Geometry check sheet. Reference: the model listing, model coordinates, mm. A direction names the side the tool comes from. Coordinates: 2 decimals unless noted, no trailing zeros.
Autodesk Inventor part; units mm, degrees
ref_plane "YZ Plane" through (0, 0, 0) normal (1, 0, 0) x (0, 1, 0)
ref_plane "XZ Plane" through (0, 0, 0) normal (0, 1, 0) x (-1, 0, 0)
ref_plane "XY Plane" through (0, 0, 0) normal (0, 0, 1) x (1, 0, 0)
sketch "Эскиз1" plane through (0, 0, 0) normal (0, 0, 1) x (1, 0, 0)
  line L0 (0, 20) -> (0, 30)
  line L1 (1, 30.1228) -> (1, 72.3772)
  line L2 (0, 72.5) -> (0, 84.4165)
  line L3 (0, 84.4165) -> (15, 84.4165)
  line L4 (6, 71.3949) -> (6, 31.1051)
  line L5 (15, 20) -> (0, 20)
  line L6 (15, 30) -> (15, 20)
  line L7 (-3, 0) -> (18, 0) construction
  line L8 (0, -16.8833) -> (0, 101.2998) construction
  line L9 (15, 84.4165) -> (15, 72.5)
  line L10 (15, 72.5) -> (6, 71.3949)
  line L11 (15, 30) -> (6, 31.1051)
  line L12 (0, 30) -> (1, 30.1228)
  line L13 (0, 72.5) -> (1, 72.3772)
  point P0 (0, 0)
  point P1 (1, 77.4165)
  point P2 (7, 77.4165)
  point P3 (7, 28)
  dimension "d0" = 15
  dimension "d2" = 5
  dimension "d5" = 40
  dimension "d7" = 168.833
  dimension "d9" = 0
  dimension "d17" = 83
  dimension "d18" = 83
  dimension "d19" = 60
  dimension "d20" = 83
  dimension "d21" = 83
  dimension "d22" = 2
  dimension "d43" = 145
revolve "Вращение1" add sketch "Эскиз1" angle 360 about axis through (-10, 0, 0) along (1, 0, 0)
chamfer "Фаска1" distance 1 angle 45 2 edges at (15, -20, 0) (0, -20, 0)
fillet "Сопряжение3" radius 6 2 edges at (6, -71.3949, 0) (6, -31.1051, 0)
chamfer "Фаска2" distance 1 angle 45 1 edges at (15, -72.5, 0)
fillet "Сопряжение4" radius 6 2 edges at (1, -30.1228, 0) (1, -72.3772, 0)
chamfer "Фаска4" distance 0.5 angle 45 2 edges at (0, -84.4165, 0) (15, -84.4165, 0)
sketch "Эскиз2" plane through (15, 0, 0) normal (1, 0, 0) x (0, 0, -1)
  circle A0 centre (0, 0) radius 84.4165
  circle A1 centre (0, 0) radius 73.5
  circle A2 centre (0, 0) radius 84.4165
  line L0 (-84.4161, 0.25) -> (-78.79, 0.25)
  line L1 (-78.79, 0.25) -> (-78.79, -0.25)
  line L2 (-78.79, -0.25) -> (-84.4161, -0.25)
  line L3 (0, -118.1831) -> (0, 118.1831)
  line L4 (118.1831, 0) -> (-118.1831, 0)
  dimension "d33" = 78.79
  dimension "d34" = 0.5
extrude "Выдавливание1" cut sketch "Эскиз2" against normal through all contours L0 L1 L4 A0 | A0 L4 L1 L2
pattern_circular "Круговой массив1" count 4 over 360 about axis through (-10, 0, 0) along (1, 0, 0) of "Выдавливание1"
properties part number "Wheel"
1. Draft check along Y on faces 6 (the conical face through (0.14, 58.78, -60.09)), 7 (the flat face through (8, 0.25, -82)), 8 (the cylindrical face through (7.598, -59.034, 60.342)). Enter one of: released by +Y, released by -Y, zero draft, split by the parting line, or undercut.
Computed values:
face 6: released by +Y
face 7: undercut
face 8: released by -Y
2. Thickness scan on line 1 along Y through (x, z) = (13.5, 24); line 2 along Z through (x, y) = (10.5, 0); line 3 along Z through (x, y) = (5, 0). Record the ranges inside material, lowest first.
Computed values:
line 1: y = -80.93 to -68.22, -18.31 to 18.31, 68.22 to 80.93
line 2: z = -78.79 to -71.9, -30.6 to -20, 20 to 30.6, 71.9 to 78.79
line 3: z = -78.79 to -20, 20 to 78.79
3. Gauge pin test, flat ends, axial feed: pin 1 Ø6 at (x, y) = (10.5, 81) entering from +Z; pin 2 Ø8 at (y, z) = (58.5, 6) entering from -X; pin 3 Ø1 at (x, z) = (1.5, -45.5) entering from -Y. Record the tip position at first contact, or that the pin passes through.
Computed values:
pin 1: stops at z = 32.28
pin 2: stops at x = 1
pin 3: stops at y = -71.42
4. Access from +Z, -Z, +X, -X, +Y, -Y to the whole of each face (thin tool, end or side, straight path). Record for faces 1 (the flat face through (6, 28, -28)), 2 (the flat face through (8, 82, -0.25)), 3 (the conical face through (14.86, -60.09, 58.78)), 4 (the flat face through (15, 0, -74)), 5 (the flat face through (8, -0.25, -82)).
Computed values:
face 1: +X
face 2: +X, -X, +Y
face 3: +Z, +X, -Y
face 4: +Z, -Z, +X, +Y, -Y
face 5: -Z, +X, -X
